```python
from build123d import *

# Parameters (mm, degrees)
SKETCH_2_R = 0.25
SKETCH_7_R = 0.9


with BuildPart() as part:
    # По траектории1: sweep along a path in Эскиз1
    with BuildLine(Plane(origin=(0, 0, 0), x_dir=(1, 0, 0), z_dir=(0, 1, 0))) as sweep_1_path:
        Line((-7, -2), (-7, -0.7))
        ThreePointArc((-7, -0.7), (-6.794974747, -0.205025253), (-6.3, 0))
        Line((-6.3, 0), (-0.7, 0))
        ThreePointArc((-0.7, 0), (-0.205025253, -0.205025253), (0, -0.7))
        Line((0, -0.7), (0, -2))
    # Эскиз2 → По траектории1 (sweep)
    with BuildSketch(Plane.XY.offset(2)):
        Circle(SKETCH_2_R)
    sweep(path=sweep_1_path.line)

    # По траектории2: sweep along a path in Эскиз6
    with BuildLine(Plane(origin=(0, 0, 0), x_dir=(1, 0, 0), z_dir=(0, 1, 0))) as sweep_2_path:
        Line((-5.4, 0), (-3.5, 0))
        Line((-3.5, 0), (-1.6, 0))
    # Эскиз7 → По траектории2 (sweep)
    with BuildSketch(Plane(origin=(-5.4, 0, 0), x_dir=(0, 0, -1), z_dir=(1, 0, 0))):
        Circle(SKETCH_7_R)
    sweep(path=sweep_2_path.line)


solid = part.part
```
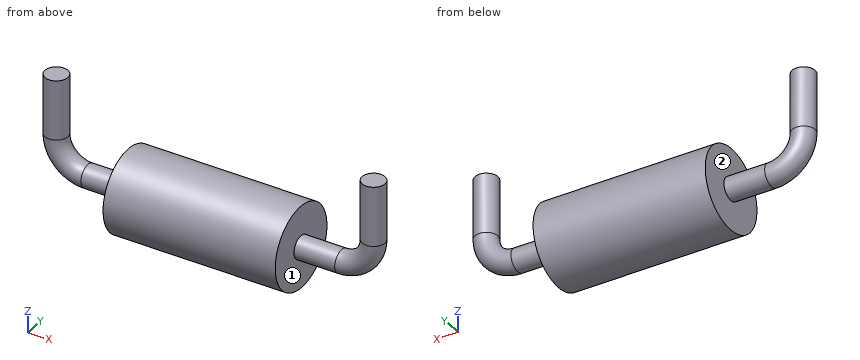
For this review, take the finished solid that the model builds, in its own axes (mm). Face numbers are marked on the shaded views. Round coordinates to 2 decimals unless told otherwise and drop trailing zeros. Loops run counter-clockwise (first coordinate to the right, second up) from the corner with the lowest first, then second, coordinate; pieces in that order, holes last.
Q1. Add section A-A on y = 0. Write out the cut boundary in (x, z).
Result sheet:
outline: (-7.25, 0.7) arc R0.95 ccw to (-6.3, -0.25) - (-5.4, -0.25) - (-5.4, -0.9) - (-1.6, -0.9) - (-1.6, -0.25) - (-0.7, -0.25) arc R0.95 ccw to (0.25, 0.7) - (0.25, 2) - (-0.25, 2) - (-0.25, 0.7) arc R0.45 cw to (-0.7, 0.25) - (-1.6, 0.25) - (-1.6, 0.9) - (-5.4, 0.9) - (-5.4, 0.25) - (-6.3, 0.25) arc R0.45 cw to (-6.75, 0.7) - (-6.75, 2) - (-7.25, 2) - close
Q2. Mouldability with a two-part tool opening along X and no side actions: class the marked faces 1 and 2 as +X half, -X half, draft (parallel to the pull), parting line (faces both ways), or undercut.
Result sheet:
face 1: undercut
face 2: undercut
Q3. To check wall thickness, follow line 1 along X through (y, z) = (-0.35, 0.1); line 2 along X through (y, z) = (0.1, 0.3); line 3 along Y through (x, z) = (-5.5, 0.15). State the ranges of each line that lie inside material, in increasing order.
Result sheet:
line 1: x = -5.4 to -1.6
line 2: x = -7.14 to -6.55, -5.4 to -1.6, -0.45 to 0.14
line 3: y = -0.2 to 0.2
Q4. Add section D-D on y = 0.35. Write out the cut boundary in (x, z), plus the area to 3 significant figures.
Result sheet:
outline: (-5.4, -0.83) - (-1.6, -0.83) - (-1.6, 0.83) - (-5.4, 0.83) - close
area: 6.30 mm2
Q5. Add section B-B on x = -2.75. Write out the cut boundary in (y, z), plus the area to 3 significant figures.
Result sheet:
outline: circle Ø1.8 at (0, 0)
area: 2.54 mm2
Q6. Insertion check: pin 1 Ø1 at (x, y) = (-5.5, 0.5) entering from +Z. The pin has a flat end and moves straight along its axis. Give the tip position at first contact, or say it passes through.
Result sheet:
pin 1: stops at z = 0.9
Q7. Add section C-C on z = 0.55. Give the number of separate pieces and of enclosed holes in the cut face, plus the area to 3 significant figures.
Result sheet:
separate pieces: 3
enclosed holes: 0
area: 5.82 mm2
